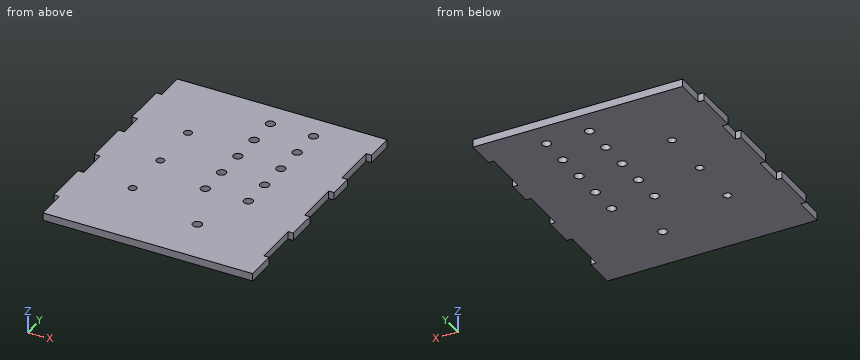
Autodesk Inventor part; units mm, degrees
ref_plane "YZ Plane" through (0, 0, 0) normal (1, 0, 0) x (0, 1, 0)
ref_plane "XZ Plane" through (0, 0, 0) normal (0, 1, 0) x (-1, 0, 0)
ref_plane "XY Plane" through (0, 0, 0) normal (0, 0, 1) x (1, 0, 0)
sketch "Sketch1" plane through (0, 0, 0) normal (0, 0, 1) x (1, 0, 0)
  line L0 (189.5387, -1221.4231) -> (189.5387, -1249.7948)
  line L1 (189.5387, -1249.7948) -> (185.3914, -1249.7948)
  line L2 (185.3914, -1227.4231) -> (26.2531, -1227.4231)
  line L3 (189.5387, -1227.4231) -> (185.3914, -1227.4231)
  line L4 (185.3914, -1249.7948) -> (185.3914, -1284.7948)
  line L5 (185.3914, -1284.7948) -> (189.5387, -1284.7948)
  line L6 (189.5387, -1284.7948) -> (189.5387, -1303.9231)
  line L7 (189.5387, -1303.9231) -> (185.3914, -1303.9231)
  line L8 (185.3914, -1303.9231) -> (185.3914, -1338.9231)
  line L9 (189.5387, -1338.9231) -> (189.5387, -1362.6731)
  line L10 (185.3914, -1338.9231) -> (189.5387, -1338.9231)
  line L11 (189.5387, -1362.6731) -> (185.3914, -1362.6731)
  line L12 (185.3914, -1362.6731) -> (185.3914, -1397.6731)
  line L13 (185.3914, -1397.6731) -> (189.5387, -1397.6731)
  line L14 (189.5387, -1397.6731) -> (189.5387, -1421.4231)
  line L15 (189.5387, -1421.4231) -> (185.3914, -1421.4231)
  line L16 (185.3914, -1421.4231) -> (26.2531, -1421.4231)
  line L17 (26.2531, -1415.4231) -> (26.2531, -1421.4231)
  line L18 (26.2531, -1421.4231) -> (26.2531, -1397.6731)
  line L19 (26.2531, -1397.6731) -> (21.9172, -1397.6731)
  line L20 (21.9172, -1397.6731) -> (21.9172, -1362.6731)
  line L21 (21.9172, -1362.6731) -> (26.2531, -1362.6731)
  line L22 (26.2531, -1362.6731) -> (26.2531, -1338.9231)
  line L23 (26.2531, -1338.9231) -> (21.9172, -1338.9231)
  line L24 (21.9172, -1338.9231) -> (21.9172, -1303.9231)
  line L25 (21.9172, -1303.9231) -> (26.2531, -1303.9231)
  line L26 (26.2531, -1303.9231) -> (26.2531, -1284.7948)
  line L27 (26.2531, -1284.7948) -> (21.9172, -1284.7948)
  line L28 (21.9172, -1284.7948) -> (21.9172, -1249.7948)
  line L29 (21.9172, -1249.7948) -> (26.2531, -1249.7948)
  line L30 (26.2531, -1249.7948) -> (26.2531, -1221.4231)
  line L31 (-159.1383, -1249.7948) -> (-159.1383, -1221.4231)
  point P0 (0, 0)
extrude "Extrusion1" add sketch "Sketch1" against normal blind 6
sketch "Sketch2" plane through (0, 0, 0) normal (0, 0, 1) x (1, 0, 0)
  circle A0 centre (109.5387, -1341.4231) radius 3.55
  line L0 (26.2531, -1421.4231) -> (189.5387, -1421.4231)
  line L1 (21.9172, -1362.6731) -> (21.9172, -1397.6731)
  line L2 (189.5387, -1421.4231) -> (189.5387, -1397.6731)
  point P0 (0, 0)
  dimension "d2" = 7.1
  dimension "d3" = 80
  dimension "d13" = 80
extrude "Extrusion2" cut sketch "Sketch2" against normal through all
pattern_linear "Rectangular Pattern1" count 5 spacing 23.5 along (0, 1, 0) count 2 spacing 33.5 along (1, 0, 0) of "Extrusion2"
sketch "Sketch3" plane through (0, 0, 0) normal (0, 0, 1) x (1, 0, 0)
  circle A0 centre (143.0387, -1341.4231) radius 3.55 construction
  circle A1 centre (109.5387, -1341.4231) radius 3.55 construction
  line L0 (143.0387, -1341.4231) -> (109.5387, -1341.4231) construction
  line L1 (126.2887, -1341.4231) -> (126.2887, -1398.6918) construction
  circle A2 centre (126.2887, -1383.9944) radius 3.6
  point P0 (0, 0)
  dimension "d14" = 7.2
extrude "Extrusion3" cut sketch "Sketch3" against normal through all
sketch "Sketch4" plane through (0, 0, 0) normal (0, 0, 1) x (1, 0, 0)
  circle A0 centre (65.2908, -1284.4231) radius 3.1
  line L0 (189.5387, -1227.4231) -> (26.2531, -1227.4231)
  circle A1 centre (65.2908, -1324.4231) radius 3.1
  circle A2 centre (65.2908, -1364.4231) radius 3.1
  line L1 (26.2531, -1421.4231) -> (189.5387, -1421.4231)
  point P0 (0, 0)
  dimension "d17" = 6.2
  dimension "d18" = 57
  dimension "d19" = 6.2
  dimension "d20" = 6.2
  dimension "d21" = 40
  dimension "d22" = 40
  dimension "d23" = 57
extrude "Extrusion4" cut sketch "Sketch4" against normal through all
properties part number "Frontpanel"
Build history of the part. All positions in model axes, mm. Give positions to 0.01 mm unless a question says otherwise; leave off trailing zeros. Order: outer loops, then holes, each group sorted by start corner. A loop starts at its lowest first (then second) coordinate and runs counter-clockwise, first axis right, second up. Notation, with made-up numbers: M 76,31 L 82,31 A32 cw 82,62 Z; hole C 25.5,-35 d10. An arc over 180 degrees is marked long. Put each result on its own line as item: value.
Item 1: Drop flat-ended pins along their axis: pin 1 Ø1.8 at (y, z) = (-1316, -4.5) entering from +X; pin 2 Ø8 at (x, y) = (63, -1256.5) entering from +Z; pin 3 Ø3 at (y, z) = (-1358, -2.5) entering from -X; pin 4 Ø5.5 at (x, y) = (109.54, -1294.42) entering from +Z. Give the stop position or say it passes through.
Results are:
pin 1: x = 185.39
pin 2: z = 0
pin 3: x = 26.25
pin 4: through
Item 2: Cut at C-C on z = -4.2. Count the separate pieces of the cut face and the enclosed holes in it, then the cut area to 3 significant figures.
Results are:
separate pieces: 1
enclosed holes: 14
area: 31,200 mm2
Item 3: Cut at A-A on x = 64.5. Write the cut outline in (y, z), then the cut area to 3 significant figures.
Results are:
outline: M -1421.42,-6 L -1367.42,-6 L -1367.42,0 L -1421.42,0 Z; M -1361.43,-6 L -1327.42,-6 L -1327.42,0 L -1361.43,0 Z; M -1321.43,-6 L -1287.42,-6 L -1287.42,0 L -1321.43,0 Z; M -1281.43,-6 L -1227.42,-6 L -1227.42,0 L -1281.43,0 Z
area: 1,060 mm2
Item 4: Wall check: probe 1 along X at (y, z) = (-1324, -0.4); probe 2 along Y at (x, z) = (63.5, -0.65); probe 3 along X at (y, z) = (-1288.5, -1.1). Give the ranges that are in metal, low to high.
Results are:
probe 1: 21.92 to 62.22, 68.36 to 185.39
probe 2: -1421.42 to -1366.95, -1361.89 to -1326.95, -1321.89 to -1286.95, -1281.89 to -1227.42
probe 3: 26.25 to 189.54
Item 5: Cut at B-B on y = -1335.5. Write the cut outline in (x, z).
Results are:
outline: M 21.92,-6 L 185.39,-6 L 185.39,0 L 21.92,0 Z
